```python
from build123d import *

# Parameters (mm, degrees)
BOSS_EXTRUDE1_DEPTH = 10


with BuildPart() as part:
    # Sketch2 → Boss-Extrude1 (new body)
    with BuildSketch(Plane(origin=(0, 0, 0), x_dir=(1, 0, 0), z_dir=(0, 1, 0))):
        with BuildLine():
            ThreePointArc((-76.2, 34.925), (-73.750256121, 26.470795103), (-66.04, 22.225))
            ThreePointArc((-66.04, 22.225), (-71.103893825, 18.75335434), (-73.66, 13.171090867))
            Line((-73.66, 13.171090867), (-73.66, -53.975))
            ThreePointArc((-73.66, -53.975), (-68.080384182, -67.445384182), (-54.61, -73.025))
            Line((-54.61, -73.025), (54.61, -73.025))
            ThreePointArc((54.61, -73.025), (68.080384182, -67.445384182), (73.66, -53.975))
            Line((73.66, -53.975), (73.66, 9.525))
            ThreePointArc((73.66, 9.525), (72.166535166, 17.2649211), (66.04, 22.225))
            ThreePointArc((66.04, 22.225), (73.750256121, 26.470795103), (76.2, 34.925))
            add(Edge.make_bspline(
                [(54.26154132, 73.334062346), (78.033661383, 68.772092229), (76.2, 34.925)],
                knots=[0, 0, 0, 1, 1, 1], degree=2))
            ThreePointArc((54.26154132, 73.334062346), (0, 79.119757765), (-54.26154132, 73.334062346))
            add(Edge.make_bspline(
                [(-54.26154132, 73.334062346), (-78.033661383, 68.772092229), (-76.2, 34.925)],
                knots=[0, 0, 0, 1, 1, 1], degree=2))
        make_face()
    extrude(amount=BOSS_EXTRUDE1_DEPTH)


solid = part.part
```
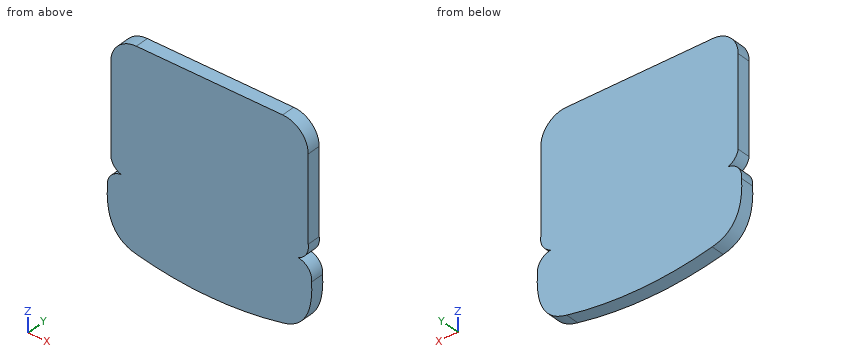
Check sheet for the modelled part. Datum: model origin and axes. Units: mm. Coordinates: 2 decimals unless noted, no trailing zeros. Write each loop counter-clockwise with the first axis right and the second up, starting at its lowest first coordinate (ties: lowest second). Pieces come first, ordered by that corner, then holes. Notation, with made-up numbers: M -24,-7.75 L 33,-7.75 A18 cw 33,14.25 Z; hole C 66,-27.75 d4. An arc over 180 degrees is marked long. Write item = value, one per line. Start each with the question number.
1. Thickness scan on probe 1 along Z at (x, y) = (-1, 2) (3 decimals); probe 2 along X at (y, z) = (6, 47.5); probe 3 along Z at (x, y) = (67.5, 8). Record the ranges inside material, lowest first.
2. Go/stop test with flat-tipped pins: pin 1 (1 mm diameter, centred on y = 2, z = 54.5, fed in from +X); pin 2 (4 mm diameter, centred on x = -5, y = 5.5, fed in from -Z); pin 3 (3 mm diameter, centred on y = 6, z = 19.5, fed in from -X). Record where each tip stops, or that it passes through.
3. Sectioned sample at B-B (x = 47). Record the cut outline in (y, z) (3 decimals).
4. Sectioned sample at A-A (z = 45). Record the cut outline in (x, y), then the cut area to 3 significant figures.
The answers:
q1.probe_1 = -79.118 to 73.025
q1.probe_2 = -73.66 to 73.66
q1.probe_3 = -66.81 to -22.48, -21.61 to 68
q2.pin_1 = 73.66
q2.pin_2 = -79.1
q2.pin_3 = -73.66
q3.outline = M 0,-74.791 L 10,-74.791 L 10,73.025 L 0,73.025 Z
q4.outline = M -73.66,0 L 73.66,0 L 73.66,10 L -73.66,10 Z
q4.area = 1,470 mm²
